Geometry check sheet. Reference: the model listing, model coordinates, mm. A direction names the side the tool comes from. Round coordinates to 2 decimals unless told otherwise and drop trailing zeros. Order: outer loops, then holes, each group sorted by start corner. A loop starts at its lowest first (then second) coordinate and runs counter-clockwise, first axis right, second up. Notation, with made-up numbers: M 56,61.25 L 89,61.25 A9 cw 89,74.25 Z; hole C 46,18 d11. An arc over 180 degrees is marked long. Answer as a JSON object with one key per item and string values. Group by question number.
```python
from build123d import *

# Parameters (mm, degrees)
BOSS_EXTRUDE1_DEPTH = 127
SKETCH3_R           = 2.5527
CUT_EXTRUDE1_DEPTH  = 137.977657098
LPATTERN1_COUNT     = 5
LPATTERN1_PITCH     = 25.4
SKETCH4_R           = 2.5527
CUT_EXTRUDE2_DEPTH  = 136.863765286
LPATTERN2_COUNT     = 5
LPATTERN2_PITCH     = 25.4


with BuildPart() as part:
    # Sketch2 → Boss-Extrude1 (new body)
    with BuildSketch(Plane(origin=(0, 0, 0), x_dir=(1, 0, 0), z_dir=(0, 1, 0))):
        Polygon((-33.319770297, 37.604825743), (-33.319770297, -0.495174257), (4.780229703, -0.495174257), (4.780229703, 2.679825743), (-30.144770297, 2.679825743), (-30.144770297, 37.604825743), align=None)
    extrude(amount=BOSS_EXTRUDE1_DEPTH)

    # Sketch3 → Cut-Extrude1 (cut, through all)
    with BuildSketch(Plane(origin=(-30.144770297, 0, 0), x_dir=(0, 0, -1), z_dir=(1, 0, 0))):
        with Locations((18.554825743, 12.7)):
            Circle(SKETCH3_R)
    cut_extrude1 = extrude(amount=-CUT_EXTRUDE1_DEPTH, mode=Mode.SUBTRACT)

    # LPattern1: Cut-Extrude1 ×5
    with Locations(*[(0, i * LPATTERN1_PITCH, 0) for i in range(1, LPATTERN1_COUNT)]):
        add(cut_extrude1, mode=Mode.SUBTRACT)

    # Sketch4 → Cut-Extrude2 (cut, through all)
    with BuildSketch(Plane(origin=(0, 0, -2.679825743), x_dir=(-1, 0, 0), z_dir=(0, 0, -1))):
        with Locations((14.269770297, 12.7)):
            Circle(SKETCH4_R)
    cut_extrude2 = extrude(amount=-CUT_EXTRUDE2_DEPTH, mode=Mode.SUBTRACT)

    # LPattern2: Cut-Extrude2 ×5
    with Locations(*[(0, i * LPATTERN2_PITCH, 0) for i in range(1, LPATTERN2_COUNT)]):
        add(cut_extrude2, mode=Mode.SUBTRACT)


solid = part.part
```
1) Set-up check for faces 1 (the flat face through (-9, 63, -2.68)), 2 (the cylindrical face through (-31.71, 11.72, -20.91)): record each of +Z, -Z, +X, -X, +Y, -Y from which the full face is reachable in a straight line by a thin tool's end or side.
2) Thickness scan on line 1 along X through (y, z) = (88.9, -1.3); line 2 along Z through (x, y) = (-26.5, 99.5); line 3 along X through (y, z) = (66, -25). Record the ranges inside material, lowest first. Write a range as [from, to].
3) Sectioned sample at D-D (z = -34). Record the boundary of the cut face in (x, y).
4) Sectioned sample at A-A (y = 88.9). Record the boundary of the cut face in (x, z).
5) Release check for a two-part mould opening along Y. For faces 3 (the flat face through (-31, 0, -10)), 4 (the flat face through (4.78, 63, -1)), 5 (the cylindrical face through (-13.716, 35.608, -1.115)) record: +Y half, -Y half, draft (parallel to the pull), parting line (faces both ways), or undercut.
6) Sectioned sample at B-B (y = 50). Record the boundary of the cut face in (x, z), then the cut area to 3 significant figures.
7) Go/stop test with flat-tipped pins: P1, Ø1, axis at x = -2, y = 64.5, coming from the -Z side; P2, Ø6, axis at y = 114.3, z = -18.55, coming from the -X side; P3, Ø3, axis at y = 73, z = -14, coming from the +X side. Record where each tip stops, or that it passes through.
8) Sectioned sample at C-C (x = -4). Record the boundary of the cut face in (y, z), then the cut area to 3 significant figures.
Final values:
{
 "1": {"face 1": "-Z, +X, +Y, -Y", "face 2": "+X, -X"},
 "2": {"line 1": "x = [-33.32, -16.82], [-11.72, 4.78]", "line 2": "z = [-2.68, 0.5]", "line 3": "x = [-33.32, -30.14]"},
 "3": {"outline": "M -33.32,0 L -30.14,0 L -30.14,127 L -33.32,127 Z"},
 "4": {"outline": "M -33.32,-37.6 L -30.14,-37.6 L -30.14,-21.11 L -33.32,-21.11 Z; M -33.32,-16 L -30.14,-16 L -30.14,-2.68 L -16.82,-2.68 L -16.82,0.5 L -33.32,0.5 Z; M -11.72,-2.68 L 4.78,-2.68 L 4.78,0.5 L -11.72,0.5 Z"},
 "5": {"face 3": "-Y half", "face 4": "draft", "face 5": "undercut"},
 "6": {"outline": "M -33.32,-37.6 L -30.14,-37.6 L -30.14,-2.68 L 4.78,-2.68 L 4.78,0.5 L -33.32,0.5 Z", "area": "232 mm^2"},
 "7": {"P1": "stops at z = -2.68", "P2": "stops at x = -33.32", "P3": "stops at x = -30.14"},
 "8": {"outline": "M 0,-2.68 L 127,-2.68 L 127,0.5 L 0,0.5 Z", "area": "403 mm^2"}
}
